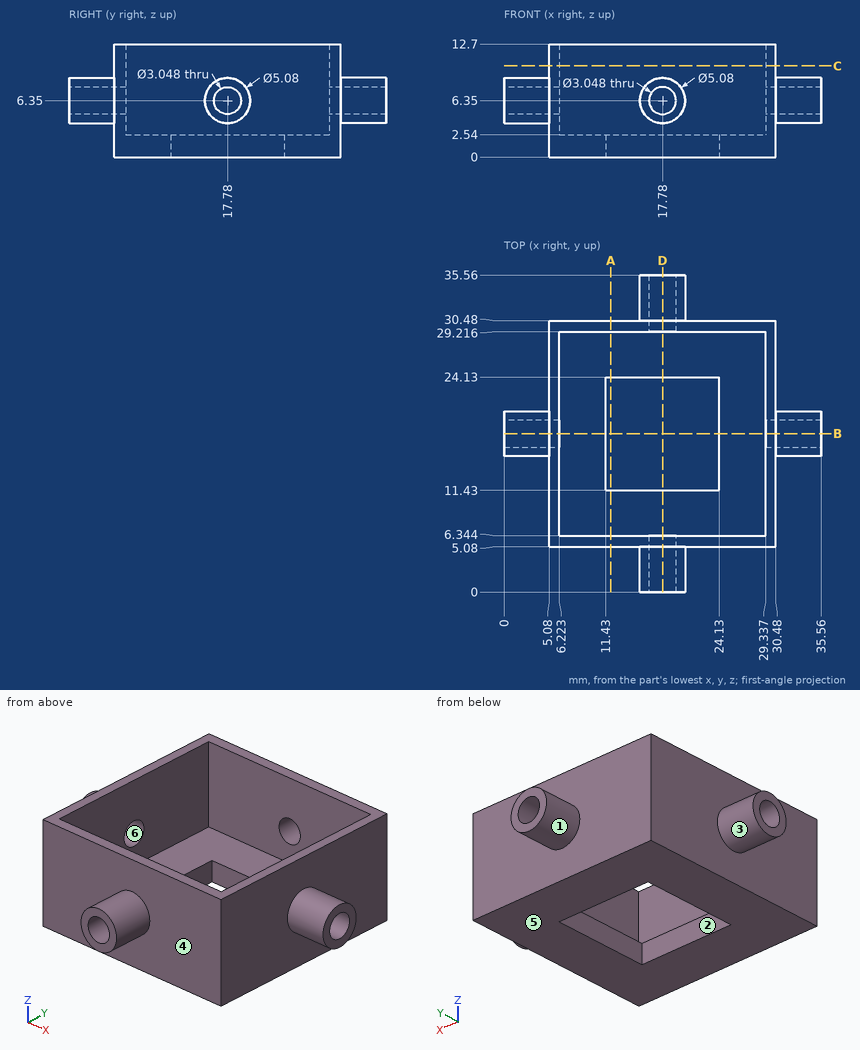
The drawing under review shows one solid part. Ordinate dimensions are in mm from its lowest x, y, z. A direction names the side the tool comes from. Round coordinates to 2 decimals unless told otherwise and drop trailing zeros. Loops run counter-clockwise (first coordinate to the right, second up) from the corner with the lowest first, then second, coordinate; pieces in that order, holes last.
Item 1: Mouldability with a two-part tool opening along Z and no side actions: class the marked faces 4, 5 and 6 as released by +Z, released by -Z, zero draft, split by the parting line, or undercut.
Determined:
face 4: zero draft
face 5: released by -Z
face 6: undercut
Item 2: Take a section at A-A (x = 12). Write out the cut boundary in (y, z) (1 decimal).
Determined:
outline: (5.1, 0) - (11.4, 0) - (11.4, 2.5) - (6.3, 2.5) - (6.3, 12.7) - (5.1, 12.7) - close; (24.1, 0) - (30.5, 0) - (30.5, 12.7) - (29.2, 12.7) - (29.2, 2.5) - (24.1, 2.5) - close
Item 3: For the marked faces 1, 2 and 3, list the 3-axis set-ups (+Z, -Z, +X, -X, +Y, -Y) from which the entire face can be reached by the end or side of a thin tool; tool diameter is ignored.
Determined:
face 1: +Y
face 2: +Z, -Z
face 3: -X
Item 4: Take a section at D-D (x = 17.78). Write out the cut boundary in (y, z) (1 decimal).
Determined:
outline: (0, 3.8) - (5.1, 3.8) - (5.1, 0) - (11.4, 0) - (11.4, 2.5) - (6.3, 2.5) - (6.3, 4.8) - (0, 4.8) - close; (0, 7.9) - (6.3, 7.9) - (6.3, 12.7) - (5.1, 12.7) - (5.1, 8.9) - (0, 8.9) - close; (24.1, 0) - (30.5, 0) - (30.5, 3.8) - (35.6, 3.8) - (35.6, 4.8) - (29.2, 4.8) - (29.2, 2.5) - (24.1, 2.5) - close; (29.2, 7.9) - (35.6, 7.9) - (35.6, 8.9) - (30.5, 8.9) - (30.5, 12.7) - (29.2, 12.7) - close
Item 5: Take a section at B-B (y = 17.78). Write out the cut boundary in (x, z).
Determined:
outline: (0, 3.81) - (5.08, 3.81) - (5.08, 0) - (11.43, 0) - (11.43, 2.54) - (6.22, 2.54) - (6.22, 4.83) - (0, 4.83) - close; (0, 7.87) - (6.22, 7.87) - (6.22, 12.7) - (5.08, 12.7) - (5.08, 8.89) - (0, 8.89) - close; (24.13, 0) - (30.48, 0) - (30.48, 3.81) - (35.56, 3.81) - (35.56, 4.83) - (29.34, 4.83) - (29.34, 2.54) - (24.13, 2.54) - close; (29.34, 7.87) - (35.56, 7.87) - (35.56, 8.89) - (30.48, 8.89) - (30.48, 12.7) - (29.34, 12.7) - close
Item 6: For line 1 (Z direction, x = 4, y = 17.78); line 2 (Y direction, x = 20.5, z = 6.75) (1 decimal); line 3 (X direction, y = 23, z = 7.75), list the stretches that pass through material, from the lowest coordinate up.
Determined:
line 1: z = 3.81 to 4.83, 7.87 to 8.89
line 2: y = 5.1 to 6.3, 29.2 to 30.5
line 3: x = 5.08 to 6.22, 29.34 to 30.48
Item 7: Take a section at C-C (z = 10.25). Write out the cut boundary in (x, y) (1 decimal).
Determined:
outline: (5.1, 5.1) - (30.5, 5.1) - (30.5, 30.5) - (5.1, 30.5) - close; hole (6.2, 6.3) - (29.3, 6.3) - (29.3, 29.2) - (6.2, 29.2) - close
Item 8: Clearance check with flat-ended pins moving along their axes: pin 1 Ø1.5 at (x, z) = (27, 3) entering from +Y; pin 2 Ø1.5 at (x, z) = (30, 7) entering from -Y; pin 3 Ø3 at (y, z) = (16.5, 1) entering from -X; pin 4 Ø2.5 at (x, z) = (17.78, 6.35) entering from +Y (3 decimals). State where each tip first meets the part, or that it passes through.
Determined:
pin 1: stops at y = 30.48
pin 2: stops at y = 5.08
pin 3: stops at x = 5.08
pin 4: passes through
